from build123d import *

# Parameters (mm, degrees)
SKETCH1_R               = 9.906
BOSS_EXTRUDE1_DEPTH     = 7.14375
SKETCH2_R               = 4.699
CUT_EXTRUDE1_DEPTH      = 8.14375
SKETCH5_W               = 1.651
SKETCH5_H               = 13.498105676
CUT_EXTRUDE3_DEPTH      = 16.3322
SKETCH6_R               = 1.143
CUT_EXTRUDE4_DEPTH      = 11.7315
CUT_EXTRUDE4_DEPTH_BACK = 10.0805
SKETCH8_R               = 3.81
CUT_EXTRUDE5_DEPTH      = 16.3322


with BuildPart() as part:
    # Sketch1 → Boss-Extrude1 (new body)
    with BuildSketch(Plane(origin=(0, 0, 0), x_dir=(1, 0, 0), z_dir=(0, 1, 0))):
        Circle(SKETCH1_R)
    extrude(amount=BOSS_EXTRUDE1_DEPTH)

    # Sketch2 → Cut-Extrude1 (cut, through all)
    with BuildSketch(Plane(origin=(0, 0, 0), x_dir=(-1, 0, 0), z_dir=(0, -1, 0))):
        Circle(SKETCH2_R)
    extrude(amount=-CUT_EXTRUDE1_DEPTH, mode=Mode.SUBTRACT)

    # Sketch5 → Cut-Extrude3 (cut)
    with BuildSketch(Plane.ZY.offset(9.906)):
        with Locations((0, 5.193192543)):
            Rectangle(SKETCH5_W, SKETCH5_H)
    extrude(amount=-CUT_EXTRUDE3_DEPTH, mode=Mode.SUBTRACT)

    # Sketch6 → Cut-Extrude4 (cut, two sides)
    with BuildSketch(Plane.XY.offset(-0.8255)) as cut_extrude4_sk:
        with Locations((-7.248732927, 3.571875)):
            Circle(SKETCH6_R)
    extrude(amount=CUT_EXTRUDE4_DEPTH, mode=Mode.SUBTRACT)
    extrude(cut_extrude4_sk.sketch, amount=-CUT_EXTRUDE4_DEPTH_BACK, mode=Mode.SUBTRACT)

    # Sketch8 → Cut-Extrude5 (cut)
    with BuildSketch(Plane(origin=(0, 0, 3.3655), x_dir=(-1, 0, 0), z_dir=(0, 0, -1))):
        with Locations((7.248732927, 3.571875)):
            Circle(SKETCH8_R)
    extrude(amount=-CUT_EXTRUDE5_DEPTH, mode=Mode.SUBTRACT)


solid = part.part
Work out the finished part from the listing and answer in its coordinate system (mm). A direction names the side the tool comes from. Round coordinates to 2 decimals unless told otherwise and drop trailing zeros. Write each loop counter-clockwise with the first axis right and the second up, starting at its lowest first coordinate (ties: lowest second). Pieces come first, ordered by that corner, then holes. Notation, with made-up numbers: (54, 38) - (83, 38) arc R14 cw to (83, 65) - close; hole circle Ø1 at (-5, -20). An arc over 180 degrees is marked (long way). Answer in a Markdown table with one row per item. Add a question column.
1. A cutting plane is placed at D-D, the plane x = 2.75. Determine the outline of the cut face in (y, z), and give its area (3 significant figures).
2. The mould has two halves that part along Y. Classify faces 4 (the flat face through (4.3, 7.144, -2.3)), 5 (the flat face through (-6, 4, 3.366)), 6 (the flat face through (6, 4, -0.826)): +Y half, -Y half, draft (parallel to the pull), parting line (faces both ways), or undercut.
3. A cutting plane is placed at B-B, the plane z = 3.75. Determine the outline of the cut face in (x, y).
4. Given pin 1 (0.5 mm diameter, centred on x = 5.5, y = 3, fed in from -Z); pin 2 (2.5 mm diameter, centred on x = -6.5, y = 3.5, fed in from +Z); pin 3 (0.5 mm diameter, centred on y = 4.5, z = 0, fed in from -X), each flat-ended and moving along its own axis, determine where each tip first touches the part or whether it passes through.
5. A cutting plane is placed at C-C, the plane z = -2. Determine the outline of the cut face in (x, y), and give its area (3 significant figures).
6. A cutting plane is placed at A-A, the plane x = 0. Determine the outline of the cut face in (y, z).
7. Find the intervals of material crossed by line 1 along X through (y, z) = (4.25, -3); line 2 along Y through (x, z) = (-7.5, -2); line 3 along Z through (x, y) = (-3.5, 6.75), in increasing order. Write a range as from..to.
8. For faces 1 (the flat face through (6, 4, 0.826)), 2 (the cylindrical face through (-0.09, 3.52, -4.7)), 3 (the cylindrical face through (-9.7, 3.5, 2)), determine the directions among +Z, -Z, +X, -X, +Y, -Y from which every point of the face is accessible in a straight line to the end or side of a thin tool.
Worked out:
| question | item | result |
|---|---|---|
| 1 | outline | (0, -9.52) - (7.14, -9.52) - (7.14, -3.81) - (0, -3.81) - close; (0, 3.81) - (7.14, 3.81) - (7.14, 9.52) - (0, 9.52) - close |
| 1 | area | 81.5 mm^2 |
| 2 | face 4 | +Y half |
| 2 | face 5 | undercut |
| 2 | face 6 | draft |
| 3 | outline | (-9.17, 0) - (-8.57, 0) arc R3.81 cw to (-9.17, 0.28) - close; (-9.17, 6.86) arc R3.81 cw to (-8.57, 7.14) - (-9.17, 7.14) - close; (-5.92, 0) - (-2.83, 0) - (-2.83, 7.14) - (-5.92, 7.14) arc R3.81 cw to start; (2.83, 0) - (9.17, 0) - (9.17, 7.14) - (2.83, 7.14) - close |
| 4 | pin 1 | z = -8.4 |
| 4 | pin 2 | z = 3.37 |
| 4 | pin 3 | x = 6.43 |
| 5 | outline | (-9.7, 0) - (-4.25, 0) - (-4.25, 7.14) - (-9.7, 7.14) - close; (4.25, 0) - (9.7, 0) - (9.7, 7.14) - (4.25, 7.14) - close; hole circle Ø2.29 at (-7.25, 3.57) |
| 5 | area | 73.8 mm^2 |
| 6 | outline | (0, -9.91) - (7.14, -9.91) - (7.14, -4.7) - (0, -4.7) - close; (0, 4.7) - (7.14, 4.7) - (7.14, 9.91) - (0, 9.91) - close |
| 7 | line 1 | -9.44..-8.17, -6.33..-3.62, 3.62..9.44 |
| 7 | line 2 | 0..2.46, 4.69..7.14 |
| 7 | line 3 | -9.27..-3.14, 3.14..9.27 |
| 8 | face 1 | -X, +Y, -Y |
| 8 | face 2 | +Y, -Y |
| 8 | face 3 | +Z, -X, +Y, -Y |
